```python
from build123d import *

# Parameters (mm, degrees)
SKETCH1_R           = 4
BOSS_EXTRUDE1_DEPTH = 3
FILLET1_R           = 10


with BuildPart() as part:
    # Sketch1 → Boss-Extrude1 (new body)
    with BuildSketch(Plane.XY):
        Polygon((-17, -7.5), (-13, -7.5), (-13, -10.5), (-8, -10.5), (-8, -7.5), (8, -7.5), (8, -10.5), (13, -10.5), (13, -7.5), (17, -7.5), (17, 7.5), (-17, 7.5), align=None)
        with Locations((0, 1.5)):
            Circle(SKETCH1_R, mode=Mode.SUBTRACT)
    extrude(amount=BOSS_EXTRUDE1_DEPTH)

    # Fillet1
    fillet1_edges = [part.edges().sort_by_distance(p)[0] for p in [
        (-17, 7.5, 1.5),
        (17, 7.5, 1.5),
    ]]
    fillet(fillet1_edges, radius=FILLET1_R)


solid = part.part
```
Part model, mm, in its own coordinate system. A direction names the side the tool comes from. Give positions to 0.01 mm unless a question says otherwise; leave off trailing zeros. Write each loop counter-clockwise with the first axis right and the second up, starting at its lowest first coordinate (ties: lowest second). Pieces come first, ordered by that corner, then holes. Notation, with made-up numbers: M 7,-6 L 23,-6 A20 cw 23,23 Z; hole C -38.5,34 d7. An arc over 180 degrees is marked long. Use CSV: the item, a comma, the result in double quotes.
Item 1: Pin check, flat tips, straight feed: P1, Ø1.5, axis at y = -9, z = 1, coming from the +X side; P2, Ø0.9, axis at x = -3, z = 2, coming from the -Y side. Stop position of each tip, or through.
Taken from the geometry:
P1,"stops at x = 13"
P2,"stops at y = -7.5"
Item 2: Drill centre lines: probe 1 along Y at (x, z) = (0, 1.15); probe 2 along Y at (x, z) = (-5.5, 1.85); probe 3 along X at (y, z) = (1.25, 1.75). Where is each one in solid material? Low to high.
Taken from the geometry:
probe 1,"y = -7.5 to -2.5, 5.5 to 7.5"
probe 2,"y = -7.5 to 7.5"
probe 3,"x = -16.27 to -3.99, 3.99 to 16.27"
Item 3: Slice it at B-B on z = 1.1. Write the cut outline in (x, y).
Taken from the geometry:
outline,"M -17,-7.5 L -13,-7.5 L -13,-10.5 L -8,-10.5 L -8,-7.5 L 8,-7.5 L 8,-10.5 L 13,-10.5 L 13,-7.5 L 17,-7.5 L 17,-2.5 A10 ccw 7,7.5 L -7,7.5 A10 ccw -17,-2.5 Z; hole C 0,1.5 d8"
Item 4: Slice it at C-C on y = 1.5. Write the cut outline in (x, z), plus the area to 3 significant figures.
Taken from the geometry:
outline,"M -16.17,0 L -4,0 L -4,3 L -16.17,3 Z; M 4,0 L 16.17,0 L 16.17,3 L 4,3 Z"
area,"73.0 mm²"
Item 5: Slice it at A-A on x = 0. Write the cut outline in (y, z), plus the area to 3 significant figures.
Taken from the geometry:
outline,"M -7.5,0 L -2.5,0 L -2.5,3 L -7.5,3 Z; M 5.5,0 L 7.5,0 L 7.5,3 L 5.5,3 Z"
area,"21.0 mm²"
Item 6: Which spindle directions (+Z, -Z, +X, -X, +Y, -Y) get a long thin tool onto all of the face, cutting with end or side? Do faces 5 (the face through (-15, -7.5, 1)), 6 (the face through (13, -9, 1)), 7 (the face through (0, -3, 3)), 8 (the face through (0, -7.5, 1)), 9 (the face through (0, 7.5, 1)). Say none if no direction does.
Taken from the geometry:
face 5,"+Z, -Z, -X, -Y"
face 6,"+Z, -Z, +X, -Y"
face 7,"+Z, +X, -X, +Y, -Y"
face 8,"+Z, -Z, -Y"
face 9,"+Z, -Z, +X, -X, +Y"
Item 7: Pull direction X, two halves, no side cores. Call faces 1 (the face through (13.99, 4.65, 1.52)), 2 (the face through (-14.15, 4.49, 1.52)), 3 (the face through (-0.867, -2.405, 1.479)), 4 (the face through (0, -3, 0)): +X half, -X half, draft (parallel to the pull), parting line (faces both ways), or undercut.
Taken from the geometry:
face 1,"+X half"
face 2,"-X half"
face 3,"undercut"
face 4,"draft"
Item 8: Slice it at D-D on x = -5. Write the cut outline in (y, z).
Taken from the geometry:
outline,"M -7.5,0 L 7.5,0 L 7.5,3 L -7.5,3 Z"
